Check sheet for the drawn part. Datum: minimum x, y, z corner. Units: mm. A direction names the side the tool comes from. Give positions to 0.01 mm unless a question says otherwise; leave off trailing zeros. Write each loop counter-clockwise with the first axis right and the second up, starting at its lowest first coordinate (ties: lowest second). Pieces come first, ordered by that corner, then holes. Notation, with made-up numbers: M 4.5,22.5 L 32.5,22.5 A3 ccw 32.5,26.5 Z; hole C 8.5,79 d11. An arc over 180 degrees is marked long. Write item = value, one per line. Start each with the question number.
1) Sectioned sample at B-B, the plane z = 51. Record the cut outline in (x, y) (1 decimal).
2) Draft check along X on the marked faces 1, 2 and 3. Enter one of: pulls with the +X half, pulls with the -X half, needs draft (parallel to the pull), parting line crosses it, or undercut.
3) Scan lines: L1, parallel to Y at x = 52, z = 53; L2, parallel to Y at x = 44, z = 39; L3, parallel to Y at x = 9.5, z = 31.5. Record each from-to range of solid material in increasing order.
4) Sectioned sample at A-A, the plane x = 9.5. Record the cut outline in (y, z).
5) Set-up check for the marked faces 4, 5 and 6: record each of +Z, -Z, +X, -X, +Y, -Y from which the full face is reachable in a straight line by a thin tool's end or side.
6) Sectioned sample at D-D, the plane z = 27.5. Record the cut outline in (x, y).
7) Sectioned sample at C-C, the plane y = 28. Record the cut outline in (x, z), then the cut area to 3 significant figures.
8) Gauge pin test, flat ends, axial feed: pin 1 (2.5 mm diameter, centred on x = 40, z = 52, fed in from +Y); pin 2 (1.5 mm diameter, centred on y = 30.5, z = 43, fed in from -X); pin 3 (10.5 mm diameter, centred on x = 8, z = 22.5, fed in from +Y). Record the tip position at first contact, or that the pin passes through.
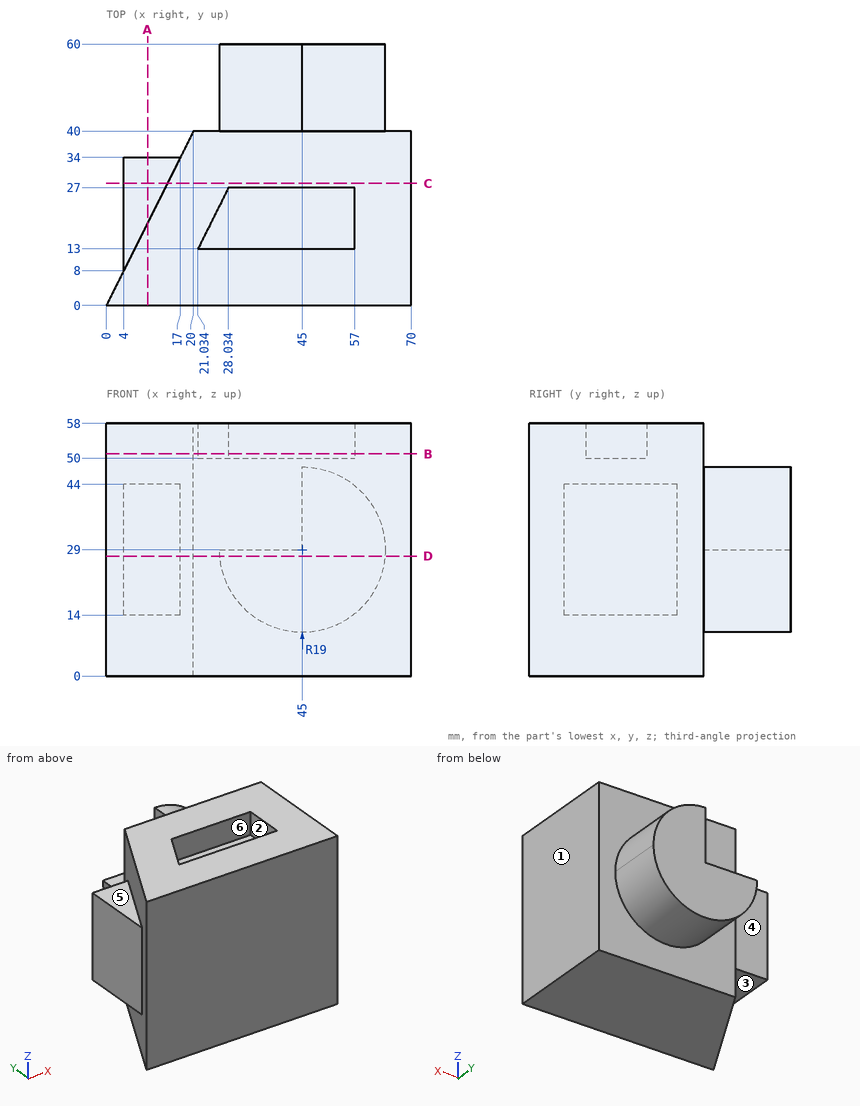
Data:
q1.outline = M 0,0 L 70,0 L 70,40 L 20,40 Z; hole M 21,13 L 57,13 L 57,27 L 28,27 Z
q2.face_1 = pulls with the +X half
q2.face_2 = undercut
q2.face_3 = needs draft
q3.L1 = 0 to 13, 27 to 40
q3.L2 = 0 to 40
q3.L3 = 0 to 34
q4.outline = M 0,0 L 19,0 L 19,14 L 34,14 L 34,44 L 19,44 L 19,58 L 0,58 Z
q5.face_4 = +Z, -Z, -X, +Y
q5.face_5 = +Z, -X, +Y
q5.face_6 = +Z
q6.outline = M 0,0 L 70,0 L 70,40 L 63.94,40 L 63.94,60 L 26.06,60 L 26.06,40 L 20,40 L 17,34 L 4,34 L 4,8 Z
q7.outline = M 4,14 L 14,14 L 14,0 L 70,0 L 70,58 L 14,58 L 14,44 L 4,44 Z
q7.area = 3,550 mm2
q8.pin_1 = 40
q8.pin_2 = 4
q8.pin_3 = 34
